```python
from build123d import *

# Parameters (mm, degrees)
F1_DEPTH = 508
F3_D     = 31.75
F5_D     = 7.9375
F7_D     = 9.525


with BuildPart() as f1:
    # F0 (on Front) → F1 (new body)
    with BuildSketch(Plane.XZ):
        Polygon((0, 3.175), (0, 0), (25.4, 0), (25.4, -38.1), (44.45, -38.1), (44.45, 0), (158.75, 0), (158.75, -38.1), (177.8, -38.1), (177.8, 0), (177.8, 3.175), align=None)
    extrude(amount=F1_DEPTH)

    # F3 (through all)
    with Locations(Plane.XY.offset(3.175)):
        with Locations((101.6, -323.85)):
            Hole(F3_D / 2)

    # F5 (through all)
    with Locations(Plane.XY.offset(3.175)):
        with Locations((101.6, -288.925), (136.525, -323.85), (101.6, -358.775), (66.675, -323.85)):
            Hole(F5_D / 2)

    # F7 (through all)
    with Locations(Plane.XY.offset(3.175)):
        with Locations((34.925, -25.4), (158.75, -25.4)):
            Hole(F7_D / 2)


solid = f1.part
```
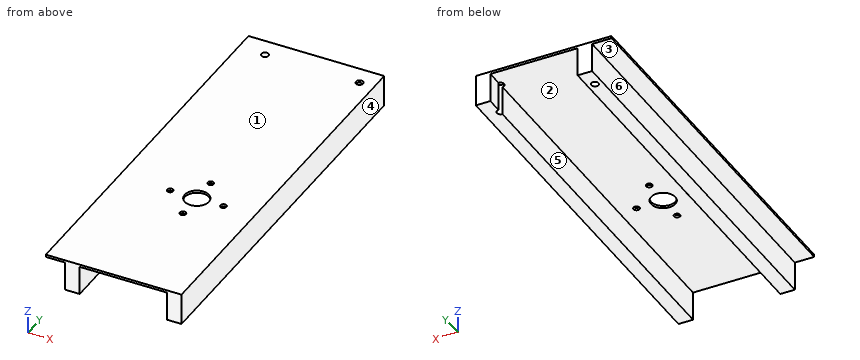
Could you check a few things on this model? Use its own coordinates, in mm. Face numbers are marked on the shaded views. A direction names the side the tool comes from. Coordinates: 2 decimals unless noted, no trailing zeros. Order: outer loops, then holes, each group sorted by start corner. A loop starts at its lowest first (then second) coordinate and runs counter-clockwise, first axis right, second up. Notation, with made-up numbers: M -9.75,42 L 30.25,42 A26 ccw 30.25,57 Z; hole C 21.5,46 d2. An arc over 180 degrees is marked long. Use a Markdown table: item, result. Add a question column.
Q1. Which directions (+Z, -Z, +X, -X, +Y, -Y) give clear straight access to the entire face, cutting with the end or side of a thin tool? Please do the marked faces 1, 2 and 3.
Q2. If I drill on L1, parallel to X at y = -25.5, z = -17.5; L2, parallel to Y at x = 101.6, z = 1.3 (3 decimals); L3, parallel to X at y = -323, z = 1, over which ranges is the centre line in solid material (lowest first)?
Q3. We'd pull the mould along X, two halves only. Please class the marked faces 4, 5 and 6: pulls with the +X half, pulls with the -X half, needs draft (parallel to the pull), parting line crosses it, or undercut.
Q4. I want a section at C-C on y = -234. List the corners of the cut face in (x, z) for me (3 decimals).
Q5. I want a section at D-D on x = 54. List the corners of the cut face in (y, z) for me (3 decimals), then the cut area to 3 significant figures.
Q6. I'm going to push flat-ended pins straight in: pin 1 (5 mm diameter, centred on x = 96.5, y = -215.5, fed in from -Z); pin 2 (11.5 mm diameter, centred on y = -157.5, z = -16, fed in from -X). Where does each tip first touch, or does it pass through?
Q7. I want a section at A-A on z = -23.5. Give the number of separate pieces and of enclosed holes in the cut face, then the cut area to 3 significant figures.
Checked values:
| question | item | result |
|---|---|---|
| 1 | face 1 | +Z, +X, -X, +Y, -Y |
| 1 | face 2 | -Z, +Y, -Y |
| 1 | face 3 | -Z, -X, +Y, -Y |
| 2 | L1 | 25.4 to 30.16, 39.69 to 44.45, 163.51 to 177.8 |
| 2 | L2 | -508 to -362.744, -354.806 to -339.725, -307.975 to -292.894, -284.956 to 0 |
| 2 | L3 | 0 to 62.8, 70.55 to 85.75, 117.45 to 132.65, 140.4 to 177.8 |
| 3 | face 4 | pulls with the +X half |
| 3 | face 5 | undercut |
| 3 | face 6 | pulls with the -X half |
| 4 | outline | M 0,0 L 25.4,0 L 25.4,-38.1 L 44.45,-38.1 L 44.45,0 L 158.75,0 L 158.75,-38.1 L 177.8,-38.1 L 177.8,3.175 L 0,3.175 Z |
| 5 | outline | M -508,0 L 0,0 L 0,3.175 L -508,3.175 Z |
| 5 | area | 1,610 mm² |
| 6 | pin 1 | z = 0 |
| 6 | pin 2 | x = 25.4 |
| 7 | separate pieces | 2 |
| 7 | enclosed holes | 1 |
| 7 | area | 19,200 mm² |
